Here's how the part is built. I have some questions about the finished solid (model axes, mm). Round coordinates to 2 decimals unless told otherwise and drop trailing zeros. Write each loop counter-clockwise with the first axis right and the second up, starting at its lowest first coordinate (ties: lowest second). Pieces come first, ordered by that corner, then holes. Notation, with made-up numbers: (-13, 6.5) - (41, 6.5) arc R17 ccw to (41, 29.5) - close; hole circle Ø5 at (14.25, 15). An arc over 180 degrees is marked (long way). Use one line per item in the form item = value. Start each with the question number.
1. I want a section at A-A, the plane z = 21. List the corners of the cut face in (x, y) for me, plus the area to 3 significant figures.
2. If I drill on line 1 along Y through (x, z) = (69, 19); line 2 along Z through (x, y) = (3.5, -4.5); line 3 along X through (y, z) = (-5, 19.5), over which ranges is the centre line in solid material (lowest first)?
3. Will this pin go through, and if not, where does the flat tip stop? pin 1 (8 mm diameter, centred on x = 45.5, z = 29.5, fed in from -Y).
4. I want a section at B-B, the plane x = 10.5. List the corners of the cut face in (y, z) for me, plus the area to 3 significant figures.
```python
from build123d import *

# Parameters (mm, degrees)
SKETCH1_W           = 78.7
SKETCH1_H           = 27.9
BOSS_EXTRUDE1_DEPTH = 38.1
SKETCH2_R           = 0.5
BOSS_EXTRUDE2_DEPTH = 10
FILLET1_R           = 1


with BuildPart() as part:
    # Sketch1 → Boss-Extrude1 (new body)
    with BuildSketch(Plane.XY):
        with Locations((39.35, 13.95)):
            Rectangle(SKETCH1_W, SKETCH1_H)
    extrude(amount=BOSS_EXTRUDE1_DEPTH)

    # Sketch2 → Boss-Extrude2 (add)
    with BuildSketch(Plane(origin=(0, 0, 0), x_dir=(-1, 0, 0), z_dir=(0, -1, 0))):
        with Locations(Location((-3.2, -4.1, 0), (0, 0, 270))):
            Circle(SKETCH2_R)
        with Locations(Location((-75.6, -4.1, 0), (0, 0, 270))):
            Circle(SKETCH2_R)
        with Locations(Location((-75.6, -34.1, 0), (0, 0, 270))):
            Circle(SKETCH2_R)
        with Locations(Location((-3.2, -19.1, 0), (0, 0, 270))):
            Circle(SKETCH2_R)
    extrude(amount=BOSS_EXTRUDE2_DEPTH)

    # Fillet1
    fillet1_edges = [part.edges().sort_by_distance(p)[0] for p in [
        (78.7, 13.95, 38.1),
        (39.35, 27.9, 38.1),
        (0, 13.95, 38.1),
        (39.35, 27.9, 0),
        (78.7, 13.95, 0),
        (39.35, 0, 0),
        (0, 13.95, 0),
        (39.35, 0, 38.1),
        (0, 27.9, 19.05),
        (78.7, 27.9, 19.05),
        (78.7, 0, 19.05),
        (0, 0, 19.05),
    ]]
    fillet(fillet1_edges, radius=FILLET1_R)


solid = part.part
```
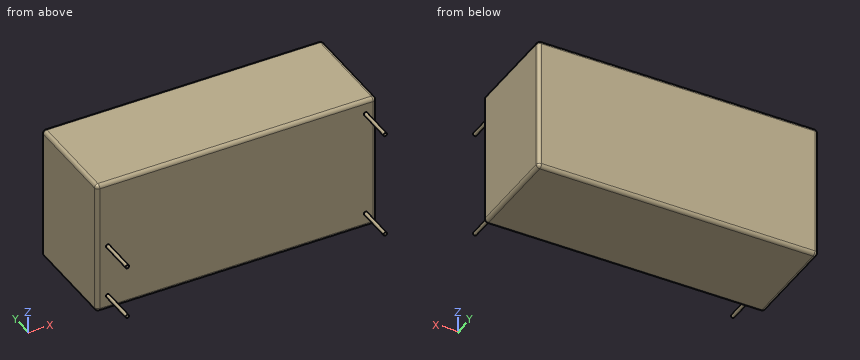
Model answer:
q1.outline = (0, 1) arc R1 ccw to (1, 0) - (77.7, 0) arc R1 ccw to (78.7, 1) - (78.7, 26.9) arc R1 ccw to (77.7, 27.9) - (1, 27.9) arc R1 ccw to (0, 26.9) - close
q1.area = 2,190 mm2
q2.line_1 = 0 to 27.9
q2.line_2 = 3.7 to 4.5, 18.7 to 19.5
q2.line_3 = 2.9 to 3.5
q3.pin_1 = 0
q4.outline = (0, 1) arc R1 ccw to (1, 0) - (26.9, 0) arc R1 ccw to (27.9, 1) - (27.9, 37.1) arc R1 ccw to (26.9, 38.1) - (1, 38.1) arc R1 ccw to (0, 37.1) - close
q4.area = 1,060 mm2
